Read the model definition and answer for the solid it produces. Units are mm, in the model's axes. A direction names the side the tool comes from. Give positions to 0.01 mm unless a question says otherwise; leave off trailing zeros. Order: outer loops, then holes, each group sorted by start corner. A loop starts at its lowest first (then second) coordinate and runs counter-clockwise, first axis right, second up. Notation, with made-up numbers: (-31, 9) - (12, 9) arc R32 cw to (12, 45) - close; hole circle Ø9 at (-7.75, -24). An arc over 180 degrees is marked (long way). Write each question's results on one line, items separated by ' | '.
from build123d import *

# Parameters (mm, degrees)
SKETCH1_R           = 10
BOSS_EXTRUDE1_DEPTH = 7
SKETCH2_R           = 10
BOSS_EXTRUDE2_DEPTH = 4
SKETCH3_R           = 7
BOSS_EXTRUDE3_DEPTH = 19
CUT_EXTRUDE5_START  = 10.2
CUT_EXTRUDE5_DEPTH  = 10.2
CHAMFER2_SIZE       = 0.5
SKETCH11_R          = 3
CUT_EXTRUDE6_DEPTH  = 36
CHAMFER3_SIZE       = 0.5


with BuildPart() as part:
    # Sketch1 → Boss-Extrude1 (new body)
    with BuildSketch(Plane.XY):
        Circle(SKETCH1_R)
    extrude(amount=-BOSS_EXTRUDE1_DEPTH)

    # Sketch2 → Boss-Extrude2 (add)
    with BuildSketch(Plane(origin=(0, 0, -7), x_dir=(-1, 0, 0), z_dir=(0, 0, -1))):
        with Locations(Location((0, 5, 0), (0, 0, 194.477512186))):
            Circle(SKETCH2_R)
    extrude(amount=BOSS_EXTRUDE2_DEPTH)

    # Sketch3 → Boss-Extrude3 (add)
    with BuildSketch(Plane(origin=(0, 0, -11), x_dir=(-1, 0, 0), z_dir=(0, 0, -1))):
        with Locations((0, 5)):
            Circle(SKETCH3_R)
    extrude(amount=BOSS_EXTRUDE3_DEPTH)

    # Sketch9 → Cut-Extrude5 (cut)
    with BuildSketch(Plane(origin=(0, 0, 0), x_dir=(1, 0, 0), z_dir=(0, 1, 0)).offset(CUT_EXTRUDE5_START)):
        with BuildLine():
            Line((2.5, 18.5), (2.5, 30))
            Line((2.5, 30), (-2.5, 30))
            Line((-2.5, 30), (-2.5, 18.5))
            ThreePointArc((-2.5, 18.5), (0, 16), (2.5, 18.5))
        make_face()
    extrude(amount=CUT_EXTRUDE5_DEPTH, mode=Mode.SUBTRACT)

    # Chamfer2
    chamfer2_edges = [part.edges().sort_by_distance(p)[0] for p in [
        (3.968626967, -0.766281297, -30),
    ]]
    chamfer(chamfer2_edges, length=CHAMFER2_SIZE)

    # Sketch11 → Cut-Extrude6 (cut, through all)
    with BuildSketch(Plane(origin=(0, 0, -30), x_dir=(-1, 0, 0), z_dir=(0, 0, -1))):
        with Locations((0, 5)):
            Circle(SKETCH11_R)
    extrude(amount=-CUT_EXTRUDE6_DEPTH, mode=Mode.SUBTRACT)

    # Chamfer3
    chamfer3_edges = [part.edges().sort_by_distance(p)[0] for p in [
        (3, 5, 0),
        (3, 5, -30),
    ]]
    chamfer(chamfer3_edges, length=CHAMFER3_SIZE)


solid = part.part
(1) The mould has two halves that part along Y. Classify faces 6 (the face through (0, 10.2, -23)), 7 (the face through (2.5, 11, -24)), 8 (the face through (0.65, 2.07, -15.2)): pulls with the +Y half, pulls with the -Y half, needs draft (parallel to the pull), parting line crosses it, or undercut.
Conclusion:
face 6: pulls with the +Y half | face 7: needs draft | face 8: undercut
(2) For faces 1 (the face through (-2.17, -9.76, -3.45)), 2 (the face through (0, 11, -16)), 3 (the face through (-3.739, -4.275, -8.972)), 4 (the face through (0, 11, -7)), 5 (the face through (0, -6, -7)), determine the directions among +Z, -Z, +X, -X, +Y, -Y from which every point of the face is accessible in a straight line to the end or side of a thin tool.
Conclusion:
face 1: +Z | face 2: -Z, +Y | face 3: -Z | face 4: +Z, +Y | face 5: -Z, -Y
(3) Section A-A (x = 0) is taken. Give the vertices of the cut face in (y, z), plus the area to 3 significant figures.
Conclusion:
outline: (-10, -7) - (-5, -7) - (-5, -11) - (-2, -11) - (-2, -29.5) - (-1.5, -30) - (1.5, -30) - (2, -29.5) - (2, -0.5) - (1.5, 0) - (-10, 0) - close; (8, -29.5) - (8.5, -30) - (10.2, -30) - (10.2, -16) - (12, -16) - (12, -11) - (15, -11) - (15, -7) - (10, -7) - (10, 0) - (8.5, 0) - (8, -0.5) - close | area: 280 mm^2
(4) Section B-B (z = -28) is taken. Give the vertices of the cut face in (x, y).
Conclusion:
outline: (-2.5, 10.2) - (-2.5, 11.54) arc R7 ccw (long way) to (2.5, 11.54) - (2.5, 10.2) - close; hole circle Ø6 at (0, 5)
(5) Consider probe 1 along Y at (x, z) = (0, -20.5); probe 2 along Y at (x, z) = (0, -11.25); probe 3 along X at (y, z) = (4.5, -22.25). Determine where each line is inside the solid, lowest interval first. Write a range as [from, to].
Conclusion:
probe 1: [-2, 2], [8, 10.2] | probe 2: [-2, 2], [8, 12] | probe 3: [-6.98, -2.96], [2.96, 6.98]
(6) Section D-D (y = -5.75) is taken. Give the vertices of the cut face in (x, z).
Conclusion:
outline: (-8.18, -7) - (8.18, -7) - (8.18, 0) - (-8.18, 0) - close
(7) Section C-C (x = -8) is taken. Give the vertices of the cut face in (y, z).
Conclusion:
outline: (-6, -7) - (-1, -7) - (-1, -11) - (11, -11) - (11, -7) - (6, -7) - (6, 0) - (-6, 0) - close
(8) Each of these flat-tipped pins is pushed along its axis until it touches: pin 1 (1 mm diameter, centred on x = 7, y = 4, fed in from +Z); pin 2 (3 mm diameter, centred on x = 1, y = -3, fed in from -Z); pin 3 (1 mm diameter, centred on y = -0.5, z = -10, fed in from -X); pin 4 (5 mm diameter, centred on x = 3, y = -5, fed in from -Z). Where does it stop, or does it pass through?
Conclusion:
pin 1: z = 0 | pin 2: z = -29.94 | pin 3: x = -8.66 | pin 4: z = -11
